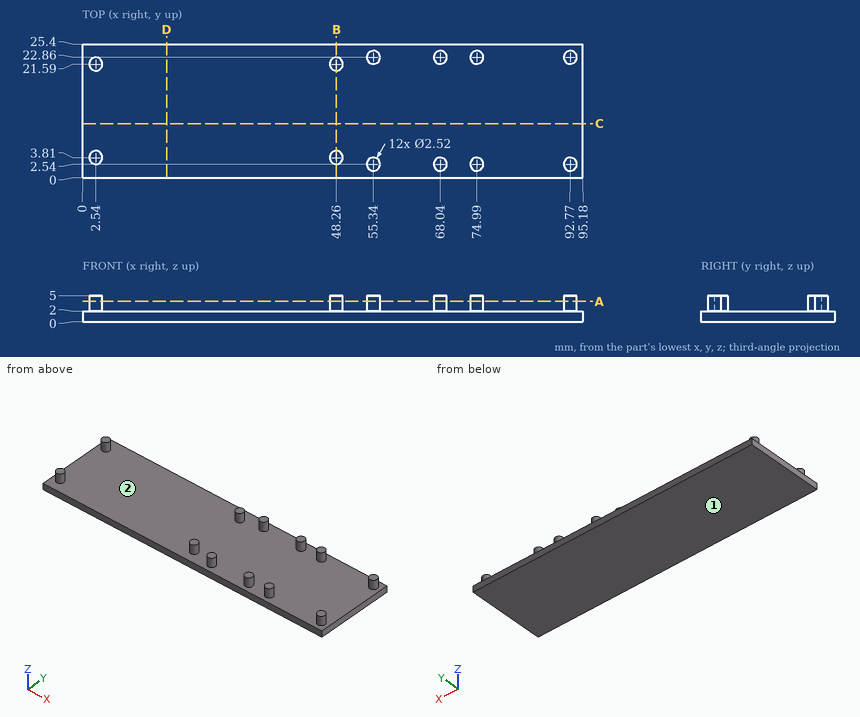
Source: three-view drawing plus pictorial views. Frame: mm from the lowest corner of the part. Give positions to 0.01 mm unless a question says otherwise; leave off trailing zeros. Write each loop counter-clockwise with the first axis right and the second up, starting at its lowest first coordinate (ties: lowest second). Pieces come first, ordered by that corner, then holes.
(1) Mould query, pull axis X, two halves, no side actions, for the marked faces 1 and 2. Classes: released by +X, released by -X, zero draft, split by the parting line, or undercut.
(2) Cut plane A-A, the plane z = 3.9. Give the number of separate pieces and of enclosed holes in the cut face, then the cut area to 3 significant figures.
(3) Cut plane B-B, the plane x = 48.26. Return loops of the section in (y, z).
(4) First-contact query: P1, Ø1.5, axis at x = 72.5, z = 3.5, coming from the +Y side; P2, Ø6, axis at x = 47.5, y = 15, coming from the +Z side; P3, Ø1.5, axis at x = 56, z = 3, coming from the -Y side. Flat tips, straight axial feed; report the tip coordinate or a pass-through.
(5) Ray query, line 1 (X direction, y = 3, z = 2.9); line 2 (X direction, y = 23.25, z = 2.7); line 3 (Z direction, x = 87, y = 7). Return the intervals inside material, ascending.
(6) Cut plane D-D, the plane x = 16. Return loops of the section in (y, z).
(7) Cut plane C-C, the plane y = 10.25. Return loops of the section in (x, z).
Values follow:
1. face 1: zero draft
1. face 2: undercut
2. separate pieces: 12
2. enclosed holes: 0
2. area: 59.9 mm2
3. outline: (0, 0) - (25.4, 0) - (25.4, 2) - (22.85, 2) - (22.85, 5) - (20.33, 5) - (20.33, 2) - (5.07, 2) - (5.07, 5) - (2.55, 5) - (2.55, 2) - (0, 2) - close
4. P1: passes through
4. P2: stops at z = 2
4. P3: stops at y = 1.28
5. line 1: x = 1.57 to 3.51, 47.29 to 49.23, 54.17 to 56.51, 66.87 to 69.21, 73.82 to 76.16, 91.6 to 93.94
5. line 2: x = 54.14 to 56.54, 66.84 to 69.24, 73.79 to 76.19, 91.57 to 93.97
5. line 3: z = 0 to 2
6. outline: (0, 0) - (25.4, 0) - (25.4, 2) - (0, 2) - close
7. outline: (0, 0) - (95.18, 0) - (95.18, 2) - (0, 2) - close
